Autodesk Inventor part; units mm, degrees
ref_plane "YZ Plane" through (0, 0, 0) normal (1, 0, 0) x (0, 1, 0)
ref_plane "XZ Plane" through (0, 0, 0) normal (0, 1, 0) x (-1, 0, 0)
ref_plane "XY Plane" through (0, 0, 0) normal (0, 0, 1) x (1, 0, 0)
sketch "Sketch1" plane through (0, 0, 0) normal (0, 0, 1) x (1, 0, 0)
  line L0 (0, 0) -> (44, 0)
  line L1 (44, 0) -> (44, 44)
  line L2 (44, 44) -> (0, 44)
  line L3 (0, 44) -> (0, 0)
  dimension "d0" = 44
  dimension "d1" = 44
extrude "Extrusion1" add sketch "Sketch1" along normal blind 4
chamfer "Chamfer1" distance 4 angle 45 4 edges at (22, 44, 4) (44, 22, 4) (22, 0, 4) (0, 22, 4)
ref_plane "Work Plane1" through (0, 22, 22) normal (0, -1, 0) x (1, 0, 0)
sketch "Sketch5" plane through (0, 22, 22) normal (0, -1, 0) x (1, 0, 0)
  line L0 (40, -18) -> (4, -18)
  line L1 (4, -18) -> (0, -22)
  line L2 (0, -22) -> (44, -22)
  line L3 (40, -18) -> (44, -22)
  line L4 (4, -18) -> (4, -22)
  line L5 (40, -18) -> (40, -22)
  line L6 (40, -22) -> (40, -21)
  line L7 (40, -21) -> (22, -18)
  line L8 (4, -22) -> (4, -21)
  line L9 (22, -18) -> (4, -21)
  dimension "d25" = 1
extrude "Extrusion4" cut sketch "Sketch5" against normal mid plane 36 contours L5 L7 L0 | L9 L4 L0
ref_plane "Work Plane2" through (22, 0, 22) normal (-1, 0, 0) x (0, -1, 0)
sketch "Sketch6" plane through (22, 0, 22) normal (-1, 0, 0) x (0, -1, 0)
  line L0 (-4, -18) -> (-40, -18)
  line L1 (-4, -18) -> (-4, -21)
  line L2 (-40, -21) -> (-40, -18)
  line L3 (-40, -21) -> (-4, -21)
  line L4 (-4, -21) -> (-22, -18)
  line L5 (-40, -18) -> (-4, -18)
  line L6 (-4, -21) -> (-40, -21)
  line L7 (-40, -21) -> (-22, -18)
  point P0 (0, -22)
extrude "Extrusion5" cut sketch "Sketch6" along normal mid plane 36 contours L1 L4 L0 | L7 L2 L0
properties part number "clear-square-inset"
Work out the finished part from the listing and answer in its coordinate system (mm). A direction names the side the tool comes from. Coordinates: 2 decimals unless noted, no trailing zeros. Loops run counter-clockwise (first coordinate to the right, second up) from the corner with the lowest first, then second, coordinate; pieces in that order, holes last. Notation, with made-up numbers: M -9,8.25 L 17,8.25 A22 cw 17,22.25 Z; hole C 22.5,50 d6. An arc over 180 degrees is marked long. Answer in a Markdown table with one row per item. Add a question column.
1. A tool of negligible diameter and unlimited length cuts with its end or side. For faces 1 (the flat face through (40, 22, 3)), 2 (the flat face through (22, 2, 2)), from which of +Z, -Z, +X, -X, +Y, -Y can it reach the whole face along a straight path? Write none if from no direction.
2. Find section A-A, the plane z = 2.7. Write down the section's boundary in (x, y), then the cut area to 3 significant figures.
3. Flat-ended cylindrical pins translate along their axes: P1, Ø1.5, axis at y = 29, z = 3, coming from the +X side; P2, Ø8, axis at x = 34, y = 19, coming from the -Z side; P3, Ø6, axis at x = 17, y = 23.5, coming from the +Z side; P4, Ø0.9, axis at y = 30, z = 3, coming from the -X side. Find the tip coordinate at first contact, or state that the pin passes through.
4. Consider L1, parallel to Y at x = 34, z = 3; L2, parallel to X at y = 16.5, z = 3.6; L3, parallel to X at y = 7.5, z = 3.8. Determine where each line is inside the solid, lowest interval first.
5. The mould has two halves that part along Y. Classify faces 3 (the flat face through (22, 42, 2)), 4 (the flat face through (22, 22, 0)), 5 (the flat face through (22.252, 10.874, 2.146)): pulls with the +Y half, pulls with the -Y half, needs draft (parallel to the pull), parting line crosses it, or undercut.
Reported:
| question | item | result |
|---|---|---|
| 1 | face 1 | +Z |
| 1 | face 2 | +Z, +X, -X, -Y |
| 2 | outline | M 2.7,2.7 L 41.3,2.7 L 41.3,41.3 L 2.7,41.3 Z; M 14.2,14.2 L 29.8,14.2 L 29.8,29.8 L 14.2,29.8 Z; hole M 4,4 L 40,4 L 40,40 L 4,40 Z |
| 2 | area | 437 mm^2 |
| 3 | P1 | stops at x = 41.75 |
| 3 | P2 | stops at z = 0 |
| 3 | P3 | stops at z = 3.67 |
| 3 | P4 | stops at x = 2.55 |
| 4 | L1 | y = 3 to 4, 40 to 41 |
| 4 | L2 | x = 3.6 to 4, 40 to 40.4 |
| 4 | L3 | x = 3.8 to 4, 40 to 40.2 |
| 5 | face 3 | pulls with the +Y half |
| 5 | face 4 | needs draft |
| 5 | face 5 | undercut |
